```python
from build123d import *

# Parameters (mm, degrees)
F0_W     = 62
F0_H     = 40
F1_DEPTH = 10
F2_R     = 1.25
F4_DEPTH = 15
F3_R     = 1.25
F5_DEPTH = 15


with BuildPart() as f1:
    # F0 (on Top) → F1 (new body)
    with BuildSketch(Plane.XY):
        Rectangle(F0_W, F0_H)
    extrude(amount=F1_DEPTH)

    # F2 (on face) → F4 (cut)
    with BuildSketch(Plane(origin=(-31, 0, 0), x_dir=(0, -1, 0), z_dir=(-1, 0, 0))):
        with Locations((10, 5)):
            Circle(F2_R)
        with Locations((-10, 5)):
            Circle(F2_R)
    extrude(amount=-F4_DEPTH, mode=Mode.SUBTRACT)

    # F3 (on face) → F5 (cut)
    with BuildSketch(Plane.YZ.offset(31)):
        with Locations((-10, 5)):
            Circle(F3_R)
        with Locations((10, 5)):
            Circle(F3_R)
    extrude(amount=-F5_DEPTH, mode=Mode.SUBTRACT)


solid = f1.part
```
Verification items for the finished model (mm, model axes). A direction names the side the tool comes from. Coordinates: 2 decimals unless noted, no trailing zeros. Loops run counter-clockwise (first coordinate to the right, second up) from the corner with the lowest first, then second, coordinate; pieces in that order, holes last. Notation, with made-up numbers: (-6, 75) - (48, 75) arc R34 ccw to (48, 112) - close; hole circle Ø6 at (-16.5, 24). An arc over 180 degrees is marked (long way). Return JSON: item names as keys, results as strings.
1. Mould release check, pull along Y, two halves, no side actions. Record for faces 1 (the flat face through (0, 20, 5)), 2 (the flat face through (-31, 0, 5)), 3 (the flat face through (-16, -10, 5)): +Y half, -Y half, draft (parallel to the pull), parting line (faces both ways), or undercut.
Established:
{"face 1": "+Y half", "face 2": "draft", "face 3": "undercut"}
2. Thickness scan on L1, parallel to Z at x = 25.5, y = -10; L2, parallel to Y at x = 23.5, z = 5.5; L3, parallel to Z at x = 26, y = 9. Record the ranges inside material, lowest first.
Established:
{"L1": "z = 0 to 3.75, 6.25 to 10", "L2": "y = -20 to -11.15, -8.85 to 8.85, 11.15 to 20", "L3": "z = 0 to 4.25, 5.75 to 10"}
3. Tool access check on faces 4 (the cylindrical face through (-23.6, 10.99, 4.24)), 5 (the flat face through (0, 0, 10)), 6 (the flat face through (16, -10, 5)). Record the directions out of +Z, -Z, +X, -X, +Y, -Y that give a thin tool (end or side, any length) a straight path to the whole face; none if there is none.
Established:
{"face 4": "-X", "face 5": "+Z, +X, -X, +Y, -Y", "face 6": "+X"}
4. Go/stop test with flat-tipped pins: pin 1 (0.8 mm diameter, centred on y = 9.5, z = 5.5, fed in from -X); pin 2 (2 mm diameter, centred on y = 10, z = 5, fed in from +X). Record where each tip stops, or that it passes through.
Established:
{"pin 1": "stops at x = -16", "pin 2": "stops at x = 16"}
5. Section check B-B, the plane y = 10. Record the boundary of the cut face in (x, z).
Established:
{"outline": "(-31, 0) - (31, 0) - (31, 3.75) - (16, 3.75) - (16, 6.25) - (31, 6.25) - (31, 10) - (-31, 10) - (-31, 6.25) - (-16, 6.25) - (-16, 3.75) - (-31, 3.75) - close"}
6. Section check A-A, the plane z = 5. Record the boundary of the cut face in (x, y), then the cut area to 3 significant figures.
Established:
{"outline": "(-31, -20) - (31, -20) - (31, -11.25) - (16, -11.25) - (16, -8.75) - (31, -8.75) - (31, 8.75) - (16, 8.75) - (16, 11.25) - (31, 11.25) - (31, 20) - (-31, 20) - (-31, 11.25) - (-16, 11.25) - (-16, 8.75) - (-31, 8.75) - (-31, -8.75) - (-16, -8.75) - (-16, -11.25) - (-31, -11.25) - close", "area": "2,330 mm2"}
